Read the model definition and answer for the solid it produces. Units are mm, in the model's axes. Face numbers are marked on the shaded views. Coordinates: 2 decimals unless noted, no trailing zeros. Loops run counter-clockwise (first coordinate to the right, second up) from the corner with the lowest first, then second, coordinate; pieces in that order, holes last. Notation, with made-up numbers: M 83,66.25 L 105,66.25 A23 ccw 105,96.25 Z; hole C -21.5,-33.75 d5. An arc over 180 degrees is marked long. Put each result on its own line as item: value.
from build123d import *

# Parameters (mm, degrees)
F1_DEPTH = 25
F2_W     = 46.5890942141
F2_H     = 40.938699618
F3_DEPTH = 5


with BuildPart() as f1:
    # F0 (on Front) → F1 (new body)
    with BuildSketch(Plane.XZ):
        with BuildLine():
            Line((-16.1972109335, 0.9067526987), (-25.7715200782, 6.687763864))
            ThreePointArc((-25.7715200782, 6.687763864), (-26.4086461718, 5.5104664675), (-26.9674355795, 4.2940318342))
            Line((-26.9674355795, 4.2940318342), (-15.7174587356, -1.9717497783))
            Line((-15.7174587356, -1.9717497783), (6.3511966728, 10.8503689989))
            ThreePointArc((6.3511966728, 10.8503689989), (5.287091796, 11.839308975), (4.1555075794, 12.7502637629))
            Line((4.1555075794, 12.7502637629), (-16.1972109335, 0.9067526987))
        make_face()
    extrude(amount=F1_DEPTH)



with BuildPart() as f1b:
    # F0 (on Front) → F1, piece 2 (new body)
    with BuildSketch(Plane.XZ):
        with BuildLine():
            Line((-16.0378590226, 6.0243331827), (-23.2363295217, 10.1388221312))
            ThreePointArc((-23.2363295217, 10.1388221312), (-24.0260011213, 9.2177770372), (-24.759702406, 8.2515536028))
            Line((-24.759702406, 8.2515536028), (-15.8774183356, 2.8789895778))
            Line((-15.8774183356, 2.8789895778), (2.4531573144, 13.8953773195))
            ThreePointArc((2.4531573144, 13.8953773195), (1.2478332365, 14.5668583693), (0, 15.1555901816))
            Line((0, 15.1555901816), (-16.0378590226, 6.0243331827))
        make_face()
    extrude(amount=F1_DEPTH)


with BuildPart() as f1c:
    # F0 (on Front) → F1, piece 3 (new body)
    with BuildSketch(Plane.XZ):
        with BuildLine():
            Line((-15.9839864927, -4.2638920279), (-27.5745631276, 2.6574631844))
            ThreePointArc((-27.5745631276, 2.6574631844), (-27.9521231277, 1.3398909811), (-28.2406369461, 0))
            Line((-28.2406369461, 0), (-16.0219292804, -7.2582247378))
            Line((-16.0219292804, -7.2582247378), (9.8358221023, 6.2114192202))
            ThreePointArc((9.8358221023, 6.2114192202), (8.7691326541, 7.944430892), (7.5355910537, 9.5629274021))
            Line((7.5355910537, 9.5629274021), (-15.9839864927, -4.2638920279))
        make_face()
    extrude(amount=F1_DEPTH)


with BuildPart() as f1d:
    # F0 (on Front) → F1, piece 4 (new body)
    with BuildSketch(Plane.XZ):
        with BuildLine():
            Line((-16.143903892, -9.4345344262), (-28.5108022498, -2.1316674104))
            ThreePointArc((-28.5108022498, -2.1316674104), (-4.7449734761, -23.3835199279), (10.6615230255, 4.528766225))
            Line((10.6615230255, 4.528766225), (-16.143903892, -9.4345344262))
        make_face()
    extrude(amount=F1_DEPTH)


with BuildPart() as f1_1:
    add(f1.part)

    add(f1b.part)  # F3 merges F1b

    add(f1c.part)  # F3 merges F1c

    add(f1d.part)  # F3 merges F1d
    # F2 (on face) → F3 (join)
    with BuildSketch(Plane(origin=(0, 0, 0), x_dir=(-1, 0, 0), z_dir=(0, 1, 0))):
        with Locations((8.2179331221, -4.6391794458)):
            Rectangle(F2_W, F2_H)
        with BuildLine():
            Line((-10.6615230255, 4.528766225), (16.143903892, -9.4345344262))
            Line((16.143903892, -9.4345344262), (28.5108022498, -2.1316674104))
            ThreePointArc((28.5108022498, -2.1316674104), (4.7449734761, -23.3835199279), (-10.6615230255, 4.528766225))
        make_face(mode=Mode.SUBTRACT)
        with BuildLine():
            Line((28.5108022498, -2.1316674104), (16.143903892, -9.4345344262))
            Line((16.143903892, -9.4345344262), (-10.6615230255, 4.528766225))
            ThreePointArc((-10.6615230255, 4.528766225), (4.7449734761, -23.3835199279), (28.5108022498, -2.1316674104))
        make_face()
    extrude(amount=F3_DEPTH)


solid = f1_1.part
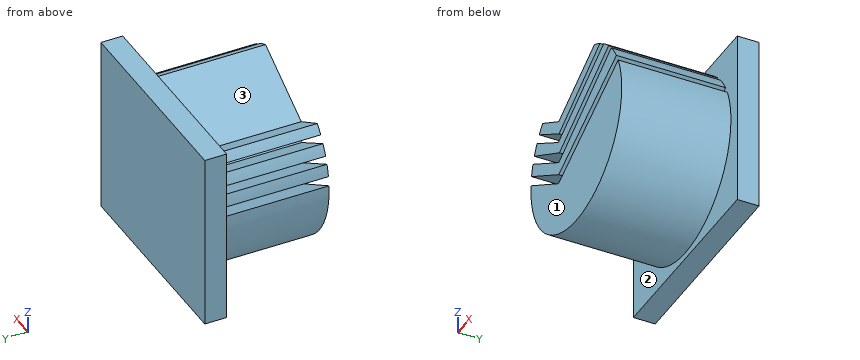
1) Given pin 1 Ø2 at (x, y) = (4, -7.5) entering from -Z; pin 2 Ø3 at (x, z) = (-3, 9.5) entering from -Y; pin 3 Ø1.5 at (x, y) = (-17, -5) entering from +Z; pin 4 Ø1 at (y, z) = (-7, -8.5) entering from +X, each flat-ended and moving along its own axis, determine where each tip first touches the part or whether it passes through.
Answer list:
pin 1: stops at z = -20.34
pin 2: stops at y = -25
pin 3: stops at z = 7
pin 4: stops at x = 11.67
2) Determine the mould class of the marked faces 1, 2 and 3 for opening direction Z: released by +Z, released by -Z, zero draft, split by the parting line, or undercut.
Answer list:
face 1: zero draft
face 2: undercut
face 3: released by +Z
3) Straight lines are drawn through the part: line 1 (Z direction, x = -3, y = -11); line 2 (Z direction, x = -10.5, y = -22.75); line 3 (Z direction, x = 4, y = -19.25). For each, find the intervals that lie inside material, in ascending order. Write a range as [from, to].
Answer list:
line 1: z = [-23.01, -2.59], [-0.47, 3.37], [5.42, 8.59], [10.62, 13.45]
line 2: z = [-23.54, -6.49], [-4.38, -1.04], [1.06, 4.22], [6.11, 9.18]
line 3: z = [-19.65, 1.06], [3.17, 7.48], [9.48, 12.66]
4) Find section B-B, the plane x = 5. Write down the section's boundary in (y, z), plus the area to 3 significant figures.
Answer list:
outline: M -25,-18.85 L 0,-18.85 L 0,-25.11 L 5,-25.11 L 5,15.83 L 0,15.83 L 0,12.08 L -25,12.08 L -25,10.07 L 0,10.07 L 0,8.07 L -25,8.07 L -25,3.69 L 0,3.69 L 0,1.58 L -25,1.58 Z
area: 875 mm^2
5) Find section A-A, the plane y = -6. Write down the section's boundary in (x, z).
Answer list:
outline: M -28.51,-2.13 A20.38 ccw long 10.66,4.53 L -16.14,-9.43 Z; M -28.24,0 L -16.02,-7.26 L 9.84,6.21 A20.46 ccw 7.54,9.56 L -15.98,-4.26 L -27.57,2.66 A20.46 ccw Z; M -26.97,4.29 L -15.72,-1.97 L 6.35,10.85 A20.46 ccw 4.16,12.75 L -16.2,0.91 L -25.77,6.69 A20.46 ccw Z; M -24.76,8.25 L -15.88,2.88 L 2.45,13.9 A20.46 ccw 0,15.16 L -16.04,6.02 L -23.24,10.14 A20.46 ccw Z
6) Find section C-C, the plane z = 3.5. Write down the section's boundary in (x, y), plus the area to 3 significant figures.
Answer list:
outline: M -31.51,0 L -25.54,0 L -25.54,-25 L -20.49,-25 L -20.49,0 L -16.9,0 L -16.9,-25 L -14.84,-25 L -14.84,0 L -11.74,0 L -11.74,-25 L -6.3,-25 L -6.3,0 L -2.78,0 L -2.78,-25 L 4.63,-25 L 4.63,0 L 8.69,0 L 8.69,-25 L 11.06,-25 L 11.06,0 L 15.08,0 L 15.08,5 L -31.51,5 Z
area: 791 mm^2
7) Find section D-D, the plane x = -20. Write down the section's boundary in (y, z).
Answer list:
outline: M -25,-19.88 L 0,-19.88 L 0,-25.11 L 5,-25.11 L 5,15.83 L 0,15.83 L 0,8.29 L -25,8.29 L -25,5.37 L 0,5.37 L 0,3.2 L -25,3.2 L -25,0.41 L 0,0.41 L 0,-1.87 L -25,-1.87 L -25,-4.9 L 0,-4.9 L 0,-7.16 L -25,-7.16 Z
